Part print with two shaded views. Sizes in mm from the minimum x, y, z corner. A direction names the side the tool comes from. Round coordinates to 2 decimals unless told otherwise and drop trailing zeros. Write each loop counter-clockwise with the first axis right and the second up, starting at its lowest first coordinate (ties: lowest second). Pieces come first, ordered by that corner, then holes. Notation, with made-up numbers: (-23, 16.5) - (5, 16.5) arc R26 cw to (5, 40.5) - close; hole circle Ø8 at (56, 30.25). An arc over 180 degrees is marked (long way). Answer as a JSON object with one key per item and string values. Group by question number.
Item 1: Slice it at C-C, the plane z = 1.5. List the corners of the cut face in (x, y), then the cut area to 3 significant figures.
Item 2: Two-plate mould, pull along X, no slides. Class the marked faces 3 and 4: +X half, -X half, draft (parallel to the pull), parting line (faces both ways), or undercut.
Item 3: Flat gauge pins, fed straight in: pin 1 (5 mm diameter, centred on x = 7.5, y = 7.5, fed in from -Z); pin 2 (4 mm diameter, centred on y = 3, z = 2, fed in from +X); pin 3 (6 mm diameter, centred on y = 3.5, z = 7, fed in from +X); pin 4 (6 mm diameter, centred on y = 9.5, z = 14, fed in from +X). Where does each tip first touch, or does it go through?
Item 4: Which spindle directions (+Z, -Z, +X, -X, +Y, -Y) get a long thin tool onto all of the face, cutting with end or side? Do the marked faces 1 and 2. Say none if no direction does.
Item 5: Probe line 1 (Z direction, x = 9, y = 5.5); line 2 (Y direction, x = 5, z = 9.5); line 3 (Y direction, x = 6, z = 3.5). List the from-to ranges inside material, lowest first. Write a range as from..to.
Item 6: Slice it at A-A, the plane y = 6. List the corners of the cut face in (x, z).
Item 7: Slice it at D-D, the plane z = 15.75. List the corners of the cut face in (x, y), then the cut area to 3 significant figures.
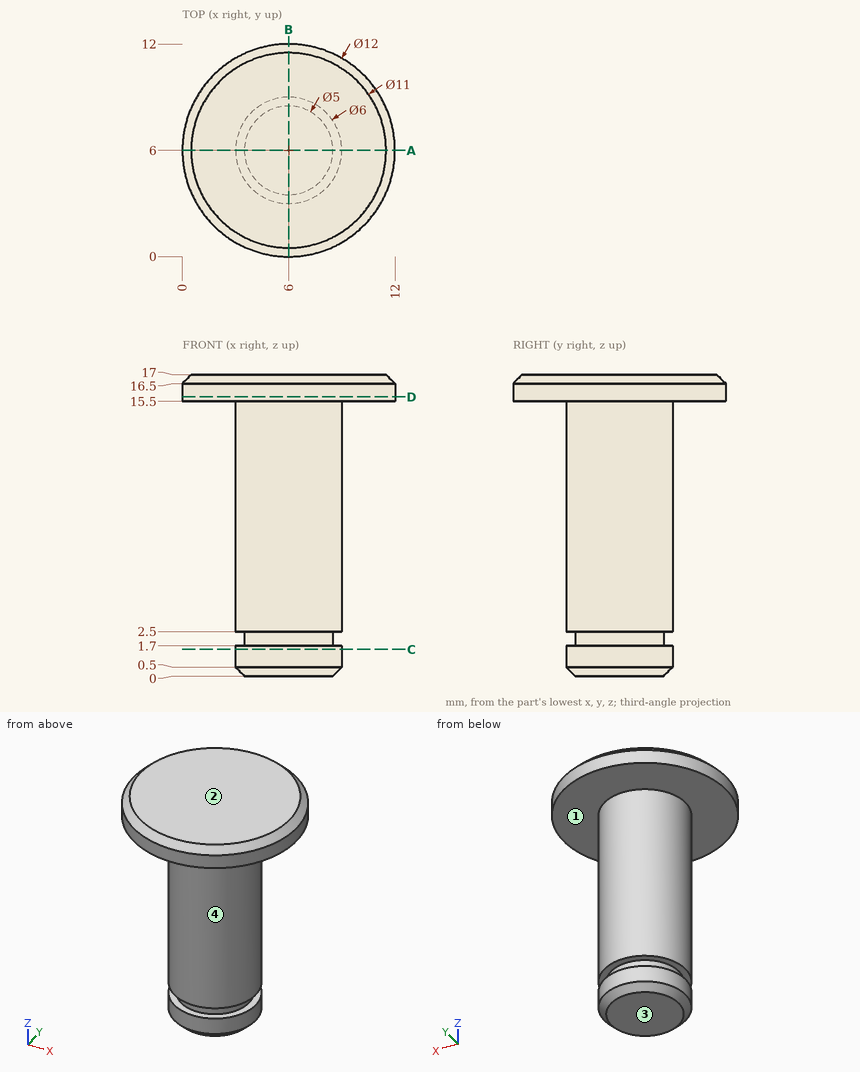
Geometry says:
{
 "1": {"outline": "circle Ø6 at (6, 6)", "area": "28.3 mm^2"},
 "2": {"face 3": "draft", "face 4": "parting line"},
 "3": {"pin 1": "stops at z = 0", "pin 2": "stops at x = 8.82", "pin 3": "stops at x = 9", "pin 4": "stops at x = 11.93"},
 "4": {"face 1": "-Z", "face 2": "+Z, +X, -X, +Y, -Y"},
 "5": {"line 1": "z = 15.5..17", "line 2": "y = 3.17..8.83", "line 3": "y = 3..9"},
 "6": {"outline": "(0, 15.5) - (3, 15.5) - (3, 2.5) - (3.5, 2.5) - (3.5, 1.7) - (3, 1.7) - (3, 0.5) - (3.5, 0) - (8.5, 0) - (9, 0.5) - (9, 1.7) - (8.5, 1.7) - (8.5, 2.5) - (9, 2.5) - (9, 15.5) - (12, 15.5) - (12, 16.5) - (11.5, 17) - (0.5, 17) - (0, 16.5) - close"},
 "7": {"outline": "circle Ø12 at (6, 6)", "area": "113 mm^2"}
}
